Build history of the part. All positions in model axes, mm. A direction names the side the tool comes from. Give positions to 0.01 mm unless a question says otherwise; leave off trailing zeros. Loops run counter-clockwise (first coordinate to the right, second up) from the corner with the lowest first, then second, coordinate; pieces in that order, holes last. Notation, with made-up numbers: M 51,-6.5 L 100,-6.5 A18 cw 100,12.5 Z; hole C -27,73 d4. An arc over 180 degrees is marked long. Answer as a JSON object with one key per item and string values. Group by question number.
1. Slice it at D-D (x = 50). List the corners of the cut face in (y, z), then the cut area to 3 significant figures.
2. Drill centre lines: line 1 along X through (y, z) = (11.5, -10); line 2 along Z through (x, y) = (100, 5); line 3 along Z through (x, y) = (60.5, -8). Where is each one in solid material? Low to high. Write a range as [from, to].
3. 3-axis set-ups, long thin cutter, end or side, ignore diameter. For faces 1 (the face through (47.5, 16, 0)), 2 (the face through (27.5, 16, 0)), 3 (the face through (0, 0, 13)), 4 (the face through (38, 19, 0)): which of +Z, -Z, +X, -X, +Y, -Y reach the whole face in a straight line?
4. Slice it at B-B (x = 89.5). List the corners of the cut face in (y, z), then the cut area to 3 significant figures.
5. Mould opens along X. For faces 5 (the face through (97.5, 0, 0)), 6 (the face through (37, 2, -17)), 7 (the face through (-27.5, 0, 0)) say: released by +X, released by -X, zero draft, split by the parting line, or undercut.
6. Slice it at A-A (z = -8). Give the number of separate pieces and of enclosed holes in the cut face, then the cut area to 3 significant figures.
7. Drop flat-ended pins along their axis: pin 1 Ø5 at (x, z) = (-25, 8) entering from +Y; pin 2 Ø2.5 at (y, z) = (16.5, 8) entering from -X. Give the stop position or say it passes through.
from build123d import *

# Parameters (mm, degrees)
F0_W     = 55
F0_H     = 34
F0_W_2   = 45
F0_H_2   = 26
F0_W_3   = 20
F1_DEPTH = 14
F2_R     = 1.5
F3_DEPTH = 30
F4_W     = 20
F4_H     = 34
F5_DEPTH = 5


with BuildPart() as f1:
    # F0 (on Front) → F1 (new body, symmetric)
    with BuildSketch(Plane.XZ):
        Rectangle(F0_W, F0_H)
        Rectangle(F0_W_2, F0_H_2, mode=Mode.SUBTRACT)
        with Locations((37.5, 0)):
            Rectangle(F0_W_3, F0_H)
        with Locations((75, 0)):
            Rectangle(F0_W, F0_H)
        with Locations((75, 0)):
            Rectangle(F0_W_2, F0_H_2, mode=Mode.SUBTRACT)
    extrude(amount=F1_DEPTH, both=True)

    # F2 (on face) → F3 (cut)
    with BuildSketch(Plane.XZ.offset(14)):
        with Locations((25, 8)):
            Circle(F2_R)
        with Locations((-25, 8)):
            Circle(F2_R)
        with Locations((-25, -8)):
            Circle(F2_R)
        with Locations((25, -8)):
            Circle(F2_R)
        with Locations((50, 8)):
            Circle(F2_R)
        with Locations((50, -8)):
            Circle(F2_R)
        with Locations((100, 8)):
            Circle(F2_R)
        with Locations((100, -8)):
            Circle(F2_R)
    extrude(amount=-F3_DEPTH, mode=Mode.SUBTRACT)

    # F4 (on face) → F5 (join)
    with BuildSketch(Plane(origin=(0, 14, 0), x_dir=(-1, 0, 0), z_dir=(0, 1, 0))):
        with Locations((-37.5, 0)):
            Rectangle(F4_W, F4_H)
    extrude(amount=F5_DEPTH)


solid = f1.part
Established:
{
 "1": {"outline": "M -14,-17 L 14,-17 L 14,-9.5 L -14,-9.5 Z; M -14,-6.5 L 14,-6.5 L 14,6.5 L -14,6.5 Z; M -14,9.5 L 14,9.5 L 14,17 L -14,17 Z", "area": "784 mm^2"},
 "2": {"line 1": "x = [-27.5, -22.5], [22.5, 52.5], [97.5, 102.5]", "line 2": "z = [-17, -9.5], [-6.5, 6.5], [9.5, 17]", "line 3": "z = [-17, -13], [13, 17]"},
 "3": {"face 1": "+Z, -Z, +X, +Y", "face 2": "+Z, -Z, -X, +Y", "face 3": "+Y, -Y", "face 4": "+Z, -Z, +X, -X, +Y"},
 "4": {"outline": "M -14,-17 L 14,-17 L 14,-13 L -14,-13 Z; M -14,13 L 14,13 L 14,17 L -14,17 Z", "area": "224 mm^2"},
 "5": {"face 5": "undercut", "face 6": "zero draft", "face 7": "released by -X"},
 "6": {"separate pieces": "7", "enclosed holes": "0", "area": "884 mm^2"},
 "7": {"pin 1": "stops at y = 14", "pin 2": "stops at x = 27.5"}
}
